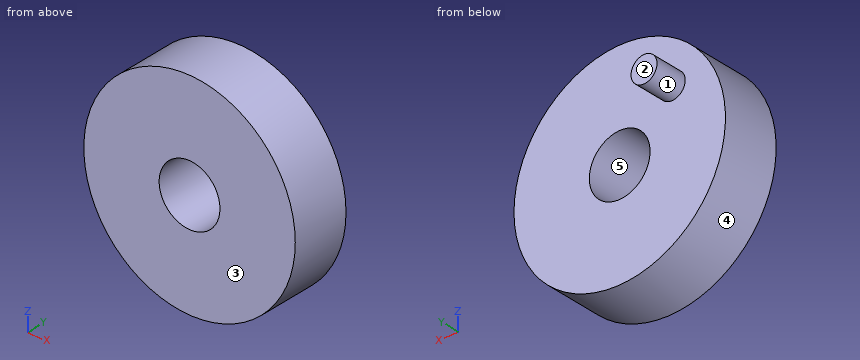
from build123d import *

# Parameters (mm, degrees)
F0_R     = 16.557582
F0_R_2   = 2.032
F0_R_3   = 4.7625
F1_DEPTH = 9.144
F2_DEPTH = 5.08
F3_DEPTH = 24.638


with BuildPart() as f1:
    # F0 (on Front) → F1 (new body)
    with BuildSketch(Plane.XZ):
        Circle(F0_R)
        with Locations((-8.22466, 7.660374)):
            Circle(F0_R_2, mode=Mode.SUBTRACT)
        Circle(F0_R_3, mode=Mode.SUBTRACT)
        Circle(F0_R_3)
        with Locations((-8.22466, 7.660374)):
            Circle(F0_R_2)
    extrude(amount=F1_DEPTH)

    # F0 (on Front) → F2 (join)
    with BuildSketch(Plane.XZ):
        with Locations((-8.22466, 7.660374)):
            Circle(F0_R_2)
    extrude(amount=-F2_DEPTH)

    # F0 (on Front) → F3 (cut)
    with BuildSketch(Plane.XZ):
        Circle(F0_R_3)
    extrude(amount=F3_DEPTH, mode=Mode.SUBTRACT)


solid = f1.part
Part model, mm, in its own coordinate system. Face numbers are marked on the shaded views. A direction names the side the tool comes from. Give positions to 0.01 mm unless a question says otherwise; leave off trailing zeros. Loops run counter-clockwise (first coordinate to the right, second up) from the corner with the lowest first, then second, coordinate; pieces in that order, holes last. Notation, with made-up numbers: M 32.5,-3.5 L 46.5,-3.5 A4 ccw 46.5,2.5 Z; hole C 48,25.5 d9. An arc over 180 degrees is marked long. Put each result on its own line as item: value. Start each with the question number.
1) Saw through at A-A (x = 0). List the corners of the cut face in (y, z), then the cut area to 3 significant figures.
2) Probe probe 1 along Z at (x, y) = (0, -6); probe 2 along Y at (x, z) = (-4.5, -4); probe 3 along Z at (x, y) = (-3.5, -2). List the from-to ranges inside material, lowest first.
3) Saw through at D-D (x = -8). List the corners of the cut face in (y, z), then the cut area to 3 significant figures.
4) 3-axis set-ups, long thin cutter, end or side, ignore diameter. For the marked faces 1 and 2: which of +Z, -Z, +X, -X, +Y, -Y reach the whole face in a straight line?
5) Saw through at B-B (z = 0). List the corners of the cut face in (x, y), then the cut area to 3 significant figures.
6) Pull direction X, two halves, no side cores. Call the marked faces 3, 4 and 5: +X half, -X half, draft (parallel to the pull), parting line (faces both ways), or undercut.
7) Saw through at C-C (y = -4.75). List the corners of the cut face in (x, z) (1 decimal), then the cut area to 3 significant figures.
8) Flat gauge pins, fed straight in: pin 1 (4 mm diameter, centred on y = -0.5, z = -7.5, fed in from +X); pin 2 (6 mm diameter, centred on y = -4, z = -11.5, fed in from -X); pin 3 (1.5 mm diameter, centred on x = -3.5, y = 3.5, fed in from +Z); pin 4 (1.5 mm diameter, centred on x = -7, y = -3, fed in from -Z). Where does each tip first touch, or does it go through?
Numbers:
1. outline: M -9.14,-16.56 L 0,-16.56 L 0,-4.76 L -9.14,-4.76 Z; M -9.14,4.76 L 0,4.76 L 0,16.56 L -9.14,16.56 Z
1. area: 216 mm^2
2. probe 1: -16.56 to -4.76, 4.76 to 16.56
2. probe 2: -9.14 to 0
2. probe 3: -16.18 to -3.23, 3.23 to 16.18
3. outline: M -9.14,-14.5 L 0,-14.5 L 0,5.64 L 5.08,5.64 L 5.08,9.68 L 0,9.68 L 0,14.5 L -9.14,14.5 Z
3. area: 286 mm^2
4. face 1: +Y
4. face 2: +Z, -Z, +X, -X, +Y
5. outline: M -16.56,-9.14 L -4.76,-9.14 L -4.76,0 L -16.56,0 Z; M 4.76,-9.14 L 16.56,-9.14 L 16.56,0 L 4.76,0 Z
5. area: 216 mm^2
6. face 3: draft
6. face 4: parting line
6. face 5: undercut
7. outline: C 0,0 d33.1; hole C 0,0 d9.5
7. area: 790 mm^2
8. pin 1: x = 15.62
8. pin 2: x = -14.21
8. pin 3: through
8. pin 4: z = -15.33
